Source: three-view drawing plus pictorial views. Frame: mm from the lowest corner of the part. A direction names the side the tool comes from. Give positions to 0.01 mm unless a question says otherwise; leave off trailing zeros. Order: outer loops, then holes, each group sorted by start corner. A loop starts at its lowest first (then second) coordinate and runs counter-clockwise, first axis right, second up. Notation, with made-up numbers: (51, -26) - (83, -26) arc R18 ccw to (83, 5) - close; hole circle Ø5 at (-18.5, -6.75). An arc over 180 degrees is marked (long way). Use one line per item in the form item = value.
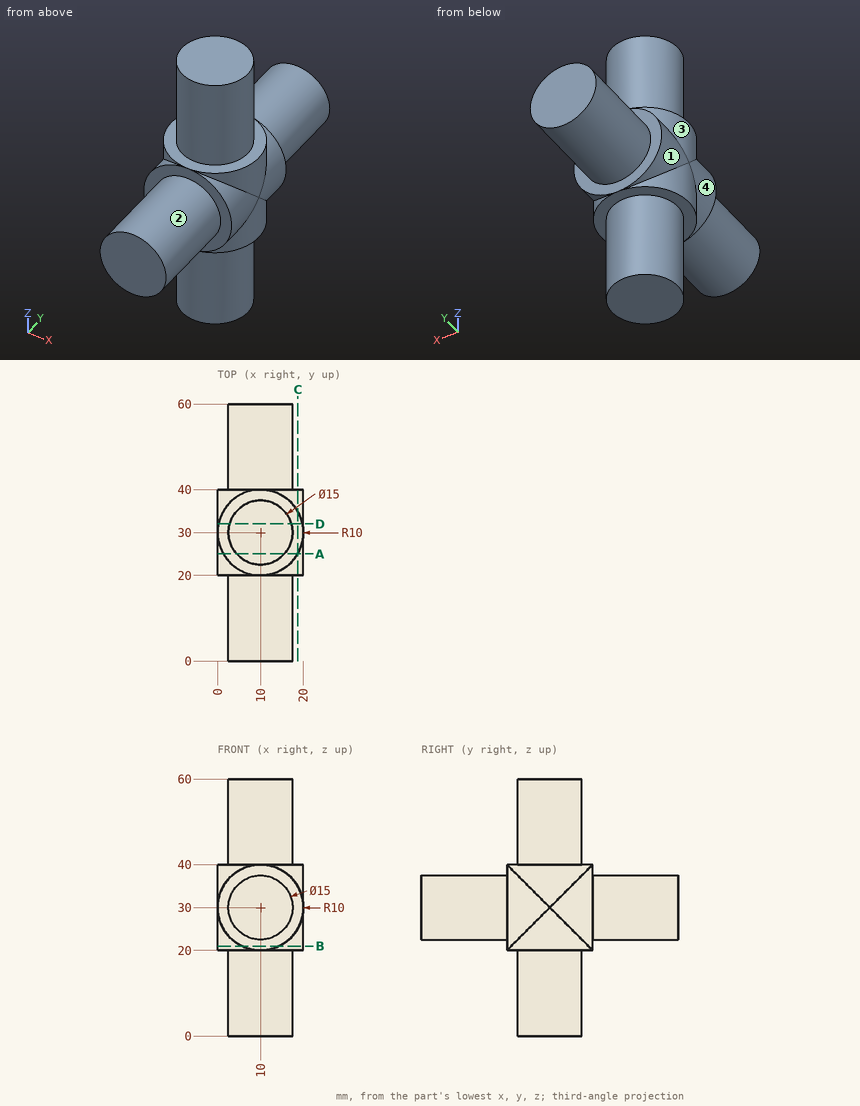
(1) Cut plane B-B on z = 21. Output: boundary loops of the cut face in (x, y).
Computed values:
outline = (5.64, 20) - (14.36, 20) - (14.36, 21) arc R10 ccw to (14.36, 39) - (14.36, 40) - (5.64, 40) - (5.64, 39) arc R10 ccw to (5.64, 21) - close
(2) Cut plane C-C on x = 18.75. Output: boundary loops of the cut face in (y, z).
Computed values:
outline = (20, 25.16) - (25.16, 25.16) - (25.16, 20) - (34.84, 20) - (34.84, 25.16) - (40, 25.16) - (40, 34.84) - (34.84, 34.84) - (34.84, 40) - (25.16, 40) - (25.16, 34.84) - (20, 34.84) - close
(3) Ray query, line 1 along Z through (x, y) = (3.5, 26); line 2 along X through (y, z) = (32, 30.5). Return the intervals inside material, ascending.
Computed values:
line_1 = 20 to 40
line_2 = 0.01 to 19.99
(4) Cut plane A-A on y = 25. Output: boundary loops of the cut face in (x, z), plus the area to 3 significant figures.
Computed values:
outline = (1.34, 20) - (4.41, 20) - (4.41, 0) - (15.59, 0) - (15.59, 20) - (18.66, 20) - (18.66, 25) arc R10 ccw to (18.66, 35) - (18.66, 40) - (15.59, 40) - (15.59, 60) - (4.41, 60) - (4.41, 40) - (1.34, 40) - (1.34, 35) arc R10 ccw to (1.34, 25) - close
area = 812 mm²
(5) Contact query for flat-ended pins moving along their axis: pin 1 Ø6 at (y, z) = (21, 37) entering from -X; pin 2 Ø2 at (x, y) = (11, 6.5) entering from +Z; pin 3 Ø5 at (x, z) = (13, 43.5) entering from -Y. Output: stop coordinate, or through.
Computed values:
pin_1 = 0.83
pin_2 = 37.5
pin_3 = 22.52
(6) Cut plane D-D on y = 32. Output: boundary loops of the cut face in (x, z).
Computed values:
outline = (0.2, 20) - (2.77, 20) - (2.77, 0) - (17.23, 0) - (17.23, 20) - (19.8, 20) - (19.8, 28) arc R10 ccw to (19.8, 32) - (19.8, 40) - (17.23, 40) - (17.23, 60) - (2.77, 60) - (2.77, 40) - (0.2, 40) - (0.2, 32) arc R10 ccw to (0.2, 28) - close
(7) Reachability of the marked faces 1, 2, 3 and 4 from +Z, -Z, +X, -X, +Y, -Y: full face, straight path, thin tool, end or side. Return the list, or none.
Computed values:
face_1 = -X, +Y
face_2 = -Y
face_3 = +Z, -X
face_4 = -X, -Y
